Check sheet for the modelled part. Datum: model origin and axes. Units: mm. Face numbers are marked on the shaded views. A direction names the side the tool comes from. Round coordinates to 2 decimals unless told otherwise and drop trailing zeros. Loops run counter-clockwise (first coordinate to the right, second up) from the corner with the lowest first, then second, coordinate; pieces in that order, holes last. Notation, with made-up numbers: (22.5, 49) -> (68.5, 49) arc R11 ccw to (68.5, 53) -> close; hole circle Ø8 at (-32.75, 27.25). An arc over 180 degrees is marked (long way). One line per question, with ' | ' between items.
```python
from build123d import *

# Parameters (mm, degrees)
F1_DEPTH = 2
F3_DEPTH = 6
F4_W     = 15
F4_H     = 3
F5_DEPTH = 15
F7_DEPTH = 1
F8_R     = 2.25
F9_DEPTH = 3.001
F10_R    = 5


with BuildPart() as f1:
    # F0 (on Right) → F1 (new body)
    with BuildSketch(Plane.YZ):
        with BuildLine():
            Line((-53.75, 25.75), (-53.75, 0))
            Line((-53.75, 0), (53.75, 0))
            Line((53.75, 0), (53.75, 25.75))
            ThreePointArc((53.75, 25.75), (45.622213, 45.372213), (26, 53.5))
            Line((26, 53.5), (-26, 53.5))
            ThreePointArc((-26, 53.5), (-45.622213, 45.372213), (-53.75, 25.75))
        make_face()
    extrude(amount=F1_DEPTH)

    # F2 (on face) → F3 (join)
    with BuildSketch(Plane(origin=(0, 0, 0), x_dir=(0, -1, 0), z_dir=(-1, 0, 0))):
        with BuildLine():
            ThreePointArc((26, 51.5), (44.208, 43.958), (51.75, 25.75))
            Line((51.75, 25.75), (51.75, 0))
            Line((51.75, 0), (53.75, 0))
            Line((53.75, 0), (53.75, 25.75))
            ThreePointArc((53.75, 25.75), (45.622213, 45.372213), (26, 53.5))
            Line((26, 53.5), (-26, 53.5))
            ThreePointArc((-26, 53.5), (-45.622213, 45.372213), (-53.75, 25.75))
            Line((-53.75, 25.75), (-53.75, 0))
            Line((-53.75, 0), (-51.75, 0))
            Line((-51.75, 0), (-51.75, 25.75))
            ThreePointArc((-51.75, 25.75), (-44.208, 43.958), (-26, 51.5))
            Line((-26, 51.5), (26, 51.5))
        make_face()
    extrude(amount=F3_DEPTH)

    # F4 (on face) → F5 (join)
    with BuildSketch(Plane(origin=(0, 0, 0), x_dir=(0, -1, 0), z_dir=(-1, 0, 0))):
        with Locations((0, 1.5)):
            Rectangle(F4_W, F4_H)
        with Locations((-46.25, 1.5)):
            Rectangle(F4_W, F4_H)
        with Locations((46.25, 1.5)):
            Rectangle(F4_W, F4_H)
    extrude(amount=F5_DEPTH)

    # F6 (on Front) → F7 (join, symmetric)
    with BuildSketch(Plane.XZ):
        Polygon((0, 18), (-6, 3), (0, 3), align=None)
    extrude(amount=F7_DEPTH, both=True)

    # F8 (on face) → F9 (cut, through all)
    with BuildSketch(Plane.XY.offset(3)):
        with Locations((-10, 48.75)):
            Circle(F8_R)
        with Locations((-10, 0)):
            Circle(F8_R)
        with Locations((-10, -48.75)):
            Circle(F8_R)
    extrude(amount=-F9_DEPTH, mode=Mode.SUBTRACT)

    # F10
    f10_edges = [f1.edges().sort_by_distance(p)[0] for p in [
        (-15, -53.75, 1.5),
        (-15, 53.75, 1.5),
        (-15, 38.75, 1.5),
        (-15, 7.5, 1.5),
        (-15, -7.5, 1.5),
        (-15, -38.75, 1.5),
    ]]
    fillet(f10_edges, radius=F10_R)


solid = f1.part
```
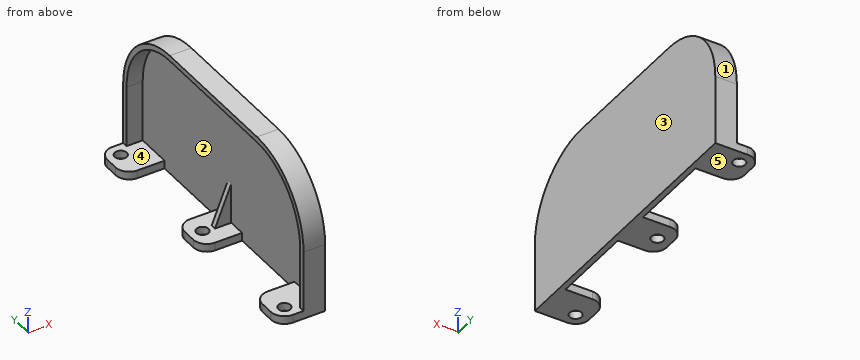
(1) Scan lines: probe 1 along Y at (x, z) = (-1.75, 2.5); probe 2 along Y at (x, z) = (-10, 1.8); probe 3 along Z at (x, y) = (-8, 41). Record each from-to range of solid material in increasing order.
Answer:
probe 1: y = -53.75 to -38.75, -7.5 to 7.5, 38.75 to 53.75 | probe 2: y = -53.75 to -51, -46.5 to -38.75, -7.5 to -2.25, 2.25 to 7.5, 38.75 to 46.5, 51 to 53.75 | probe 3: z = 0 to 3
(2) Sectioned sample at A-A, the plane y = 0. Record the cut outline in (x, z).
Answer:
outline: (-15, 0) -> (-12.25, 0) -> (-12.25, 3) -> (-15, 3) -> close; (-7.75, 0) -> (2, 0) -> (2, 53.5) -> (-6, 53.5) -> (-6, 51.5) -> (0, 51.5) -> (0, 18) -> (-6, 3) -> (-7.75, 3) -> close
(3) Mould release check, pull along Y, two halves, no side actions. Record for the marked faces 1, 2 and 3: +Y half, -Y half, draft (parallel to the pull), parting line (faces both ways), or undercut.
Answer:
face 1: +Y half | face 2: undercut | face 3: draft
(4) Sectioned sample at C-C, the plane z = 21. Record the cut outline in (x, y).
Answer:
outline: (-6, -53.75) -> (2, -53.75) -> (2, 53.75) -> (-6, 53.75) -> (-6, 51.75) -> (0, 51.75) -> (0, -51.75) -> (-6, -51.75) -> close
(5) Set-up check for the marked faces 4 and 5: record each of +Z, -Z, +X, -X, +Y, -Y from which the full face is reachable in a straight line by a thin tool's end or side.
Answer:
face 4: -X | face 5: -Z, +X, -X, +Y, -Y
(6) Sectioned sample at B-B, the plane x = -2. Record the cut outline in (y, z).
Answer:
outline: (-53.75, 0) -> (-38.75, 0) -> (-38.75, 3) -> (-51.75, 3) -> (-51.75, 25.75) arc R25.75 cw to (-26, 51.5) -> (26, 51.5) arc R25.75 cw to (51.75, 25.75) -> (51.75, 3) -> (38.75, 3) -> (38.75, 0) -> (53.75, 0) -> (53.75, 25.75) arc R27.75 ccw to (26, 53.5) -> (-26, 53.5) arc R27.75 ccw to (-53.75, 25.75) -> close; (-7.5, 0) -> (7.5, 0) -> (7.5, 3) -> (1, 3) -> (1, 13) -> (-1, 13) -> (-1, 3) -> (-7.5, 3) -> close
(7) Go/stop test with flat-tipped pins: pin 1 (7 mm diameter, centred on x = -10, y = -48.75, fed in from +Z); pin 2 (2 mm diameter, centred on y = 28.5, z = 21, fed in from -X); pin 3 (10 mm diameter, centred on x = -1, z = 35.5, fed in from +Y). Record where each tip stops, or that it passes through.
Answer:
pin 1: stops at z = 3 | pin 2: stops at x = 0 | pin 3: stops at y = 53.34
(8) Sectioned sample at D-D, the plane y = 15. Record the cut outline in (x, z).
Answer:
outline: (-6, 51.5) -> (0, 51.5) -> (0, 0) -> (2, 0) -> (2, 53.5) -> (-6, 53.5) -> close
